Check sheet for the modelled part. Datum: model origin and axes. Units: mm. Give positions to 0.01 mm unless a question says otherwise; leave off trailing zeros. Loops run counter-clockwise (first coordinate to the right, second up) from the corner with the lowest first, then second, coordinate; pieces in that order, holes last. Notation, with made-up numbers: M 55,-7 L 68,-7 A26 cw 68,7 Z; hole C -22,-31 d8. An arc over 180 degrees is marked long. Write each question's results on one line, items separated by ' | '. Start each with the question number.
1. Go/stop test with flat-tipped pins: pin 1 (2 mm diameter, centred on x = 4.5, y = 29, fed in from +Z); pin 2 (5 mm diameter, centred on y = 12, z = 4.5, fed in from -X); pin 3 (1.5 mm diameter, centred on y = 25, z = -3, fed in from +X). Record where each tip stops, or that it passes through.
2. Sectioned sample at A-A on y = 15. Record the cut outline in (x, z).
3. Material ranges on line 1 along Y through (x, z) = (-7.25, 3.25); line 2 along Z through (x, y) = (-3.5, 35); line 3 along Z through (x, y) = (0, 37.5), recorded low to high.
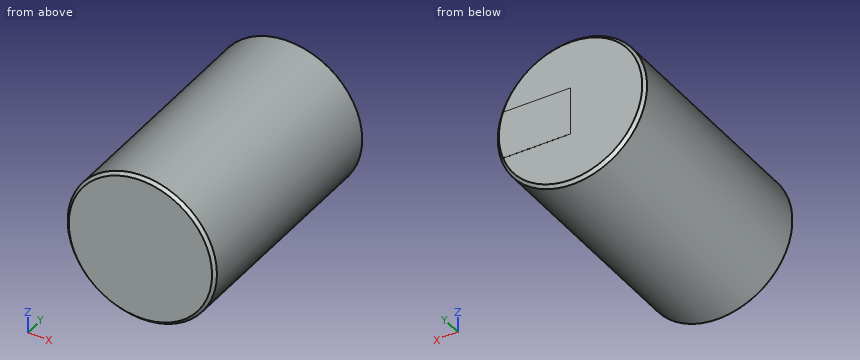
```python
from build123d import *

# Parameters (mm, degrees)
SKETCH1_R           = 12.5
BOSS_EXTRUDE1_DEPTH = 40
CHAMFER1_SIZE       = 0.5
BOSS_EXTRUDE2_DEPTH = 0.01


with BuildPart() as part:
    # Sketch1 → Boss-Extrude1 (new body)
    with BuildSketch(Plane(origin=(0, 0, 0), x_dir=(1, 0, 0), z_dir=(0, 1, 0))):
        Circle(SKETCH1_R)
    extrude(amount=BOSS_EXTRUDE1_DEPTH)

    # Chamfer1
    chamfer1_edges = [part.edges().sort_by_distance(p)[0] for p in [
        (-12.5, 0, 0),
        (-12.5, 40, 0),
    ]]
    chamfer(chamfer1_edges, length=CHAMFER1_SIZE)

    # Sketch2 → Boss-Extrude2 (add)
    with BuildSketch(Plane(origin=(0, 40, 0), x_dir=(1, 0, 0), z_dir=(0, 1, 0))):
        with BuildLine():
            Line((11.313708499, 4), (0, 4))
            Line((0, 4), (0, -4))
            Line((0, -4), (11.313708499, -4))
            ThreePointArc((11.313708499, -4), (12, 0), (11.313708499, 4))
        make_face()
    extrude(amount=BOSS_EXTRUDE2_DEPTH)


solid = part.part
```
Output values:
1) pin 1: z = 12 | pin 2: x = -12.34 | pin 3: x = 12.3
2) outline: C 0,0 d25
3) line 1: 0 to 40 | line 2: -12 to 12 | line 3: -12.5 to 12.5
